Here's the drawing with two shaded views (mm, measured from the low corner). I have some questions. A direction names the side the tool comes from. Round coordinates to 2 decimals unless told otherwise and drop trailing zeros. Loops run counter-clockwise (first coordinate to the right, second up) from the corner with the lowest first, then second, coordinate; pieces in that order, holes last. Notation, with made-up numbers: M 11.25,77 L 43.25,77 A30 ccw 43.25,109 Z; hole C 83.25,63.25 d9. An arc over 180 degrees is marked long. One line per item, written item: value. Start each with the question number.
Q1. Imagine slicing it at B-B (x = 3.25). Please give me the cut outline in (y, z), then the cut area to 3 significant figures.
Q2. Imagine slicing it at D-D (y = 18). Please give me the cut outline in (x, z), then the cut area to 4 significant figures.
Q3. Thinking about a two-plate mould opening in Z: for the marked faces 6, 7 and 8, which applies, released by +Z, released by -Z, zero draft, split by the parting line, or undercut?
Q4. I'm going to push flat-ended pins straight in: pin 1 Ø2 at (x, y) = (4, 23) entering from -Z; pin 2 Ø2 at (x, z) = (2, 5.5) entering from +Y; pin 3 Ø2 at (x, y) = (4, 27.5) entering from +Z. Where does each tip first touch, or does it pass through?
Q5. Please list where these lines run through material, in increasing order: line 1 along Z through (x, y) = (4.5, 26.5); line 2 along Y through (x, z) = (1.5, 3.5); line 3 along Z through (x, y) = (2.5, 22).
Q6. Imagine slicing it at C-C (z = 28). Please give me the cut outline in (x, y).
Q7. Which directions (+Z, -Z, +X, -X, +Y, -Y) give clear straight access to the entire face, cutting with the end or side of a thin tool? Please do the marked faces 1, 2, 3, 4 and 5.
Q8. Imagine slicing it at A-A (y = 28). Please give me the cut outline in (x, z), then the cut area to 3 significant figures.
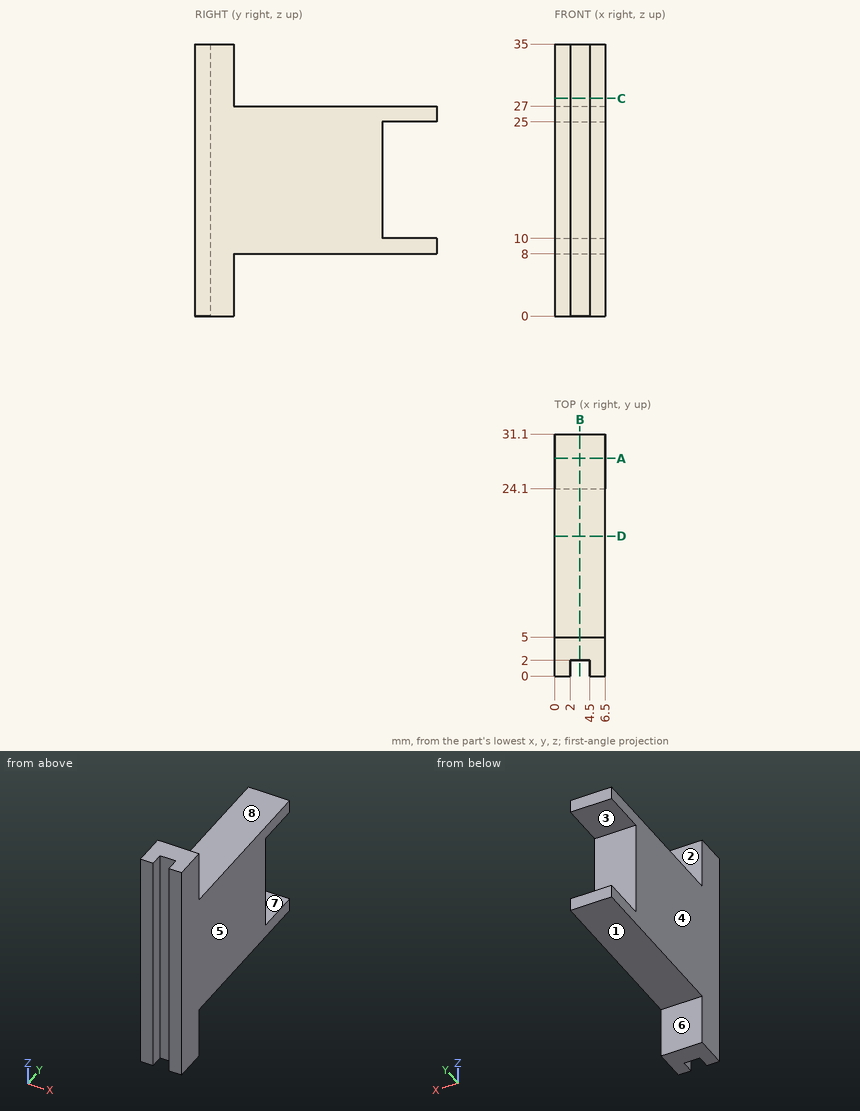
Report:
1. outline: M 2,0 L 5,0 L 5,8 L 31.1,8 L 31.1,10 L 24.1,10 L 24.1,25 L 31.1,25 L 31.1,27 L 5,27 L 5,35 L 2,35 Z
1. area: 496 mm²
2. outline: M 0,8 L 6.5,8 L 6.5,27 L 0,27 Z
2. area: 123.5 mm²
3. face 6: zero draft
3. face 7: undercut
3. face 8: released by +Z
4. pin 1: stops at z = 8
4. pin 2: stops at y = 5
4. pin 3: stops at z = 27
5. line 1: z = 8 to 10, 25 to 27
5. line 2: y = 0 to 5
5. line 3: z = 8 to 27
6. outline: M 0,0 L 2,0 L 2,2 L 4.5,2 L 4.5,0 L 6.5,0 L 6.5,5 L 0,5 Z
7. face 1: -Z, +X, -X, +Y
7. face 2: +Z, +X, -X, +Y
7. face 3: +X, -X, +Y
7. face 4: +Z, -Z, -X, +Y, -Y
7. face 5: +Z, -Z, +X, +Y, -Y
8. outline: M 0,8 L 6.5,8 L 6.5,10 L 0,10 Z; M 0,25 L 6.5,25 L 6.5,27 L 0,27 Z
8. area: 26.0 mm²
